For this review, take the finished solid that the model builds, in its own axes (mm). A direction names the side the tool comes from. Coordinates: 2 decimals unless noted, no trailing zeros. Order: outer loops, then holes, each group sorted by start corner. A loop starts at its lowest first (then second) coordinate and runs counter-clockwise, first axis right, second up. Notation, with made-up numbers: (-12.75, -10.75) -> (10.25, -10.75) arc R31 ccw to (10.25, 16.25) -> close; hole circle Ø7 at (86, 41). An arc over 180 degrees is marked (long way). Return JSON: item names as keys, results as strings. Group by question number.
Item 1: For line 1 along Y through (x, z) = (63.25, 10.3); line 2 along Z through (x, y) = (61.8, 84.5), list the stretches that pass through material, from the lowest coordinate up.
Item 2: Draft analysis for pull direction Y (two halves, no side actions). For faces 3 (the flat face through (63, 90, 9)), 4 (the flat face through (63, 91, 11)), 5 (the flat face through (63, 89, 10)), 6 (the flat face through (63, 82, 10)), state which applies: +Y half, -Y half, draft (parallel to the pull), parting line (faces both ways), or undercut.
Item 3: Take a section at B-B (x = 62.65). Write out the cut boundary in (y, z), then the cut area to 3 significant figures.
Item 4: Machinability: for faces 1 (the flat face through (63, 86, 10.5)), 2 (the flat face through (61.5, 85, 11)), which of the approach directions +Z, -Z, +X, -X, +Y, -Y give a long, thin tool a straight path to every point of the face, cutting with its end or side? Answer none if there is none.
Item 5: Take a section at C-C (y = 83.75). Write out the cut boundary in (x, z).
Item 6: Take a section at A-A (z = 9.2). Write out the cut boundary in (x, y).
```python
from build123d import *

# Parameters (mm, degrees)
BOX028_W     = 3
BOX028_H     = 7
BOX028_DEPTH = 2
BOX029_W     = 3
BOX029_H     = 2
BOX029_DEPTH = 3.5
BOX030_W     = 3
BOX030_H     = 2
BOX030_DEPTH = 3.5


with BuildPart() as obj1:
    # Box028 → Box028 (new body)
    with BuildSketch(Plane(origin=(17.5, 39, 10), x_dir=(1, 0, 0), z_dir=(0, 0, 1))):
        with Locations((1.5, 3.5)):
            Rectangle(BOX028_W, BOX028_H)
    extrude(amount=BOX028_DEPTH)


with BuildPart() as obj2:
    # Box029 → Box029 (new body)
    with BuildSketch(Plane(origin=(17.5, 46, 8.5), x_dir=(1, 0, 0), z_dir=(0, 0, 1))):
        with Locations((1.5, 1)):
            Rectangle(BOX029_W, BOX029_H)
    extrude(amount=BOX029_DEPTH)


with BuildPart() as obj3:
    # Box030 → Box030 (new body)
    with BuildSketch(Plane(origin=(17.5, 37, 8.5), x_dir=(1, 0, 0), z_dir=(0, 0, 1))):
        with Locations((1.5, 1)):
            Rectangle(BOX030_W, BOX030_H)
    extrude(amount=BOX030_DEPTH)

    # Fusion028: union obj1, obj2
    add(obj1.part)
    add(obj2.part)


with BuildPart() as obj3_1:
    # Fusion028 placement: moved
    add(obj3.part.moved(Location((44, 43, 0.5))))


solid = obj3_1.part
```
Findings below:
{
 "1": {"line 1": "y = 80 to 82, 89 to 91", "line 2": "z = 10.5 to 12.5"},
 "2": {"face 3": "draft", "face 4": "+Y half", "face 5": "undercut", "face 6": "undercut"},
 "3": {"outline": "(80, 9) -> (82, 9) -> (82, 10.5) -> (89, 10.5) -> (89, 9) -> (91, 9) -> (91, 12.5) -> (80, 12.5) -> close", "area": "28.0 mm2"},
 "4": {"face 1": "-Z, +X, -X", "face 2": "+Z, -Z, -X, +Y, -Y"},
 "5": {"outline": "(61.5, 10.5) -> (64.5, 10.5) -> (64.5, 12.5) -> (61.5, 12.5) -> close"},
 "6": {"outline": "(61.5, 80) -> (64.5, 80) -> (64.5, 82) -> (61.5, 82) -> close; (61.5, 89) -> (64.5, 89) -> (64.5, 91) -> (61.5, 91) -> close"}
}
